Study the drawing (mm; zero at the part's minimum x, y, z) and answer. A direction names the side the tool comes from. Coordinates: 2 decimals unless noted, no trailing zeros. Write each loop counter-clockwise with the first axis right and the second up, starting at its lowest first coordinate (ties: lowest second). Pieces come first, ordered by that corner, then holes. Notation, with made-up numbers: (8.5, -19) -> (26.5, -19) arc R14 ccw to (26.5, -8) -> close; hole circle Ø7 at (-9.75, 20). An arc over 180 degrees is marked (long way). Write each question's results on one line, items separated by ' | '. Start each with the question number.
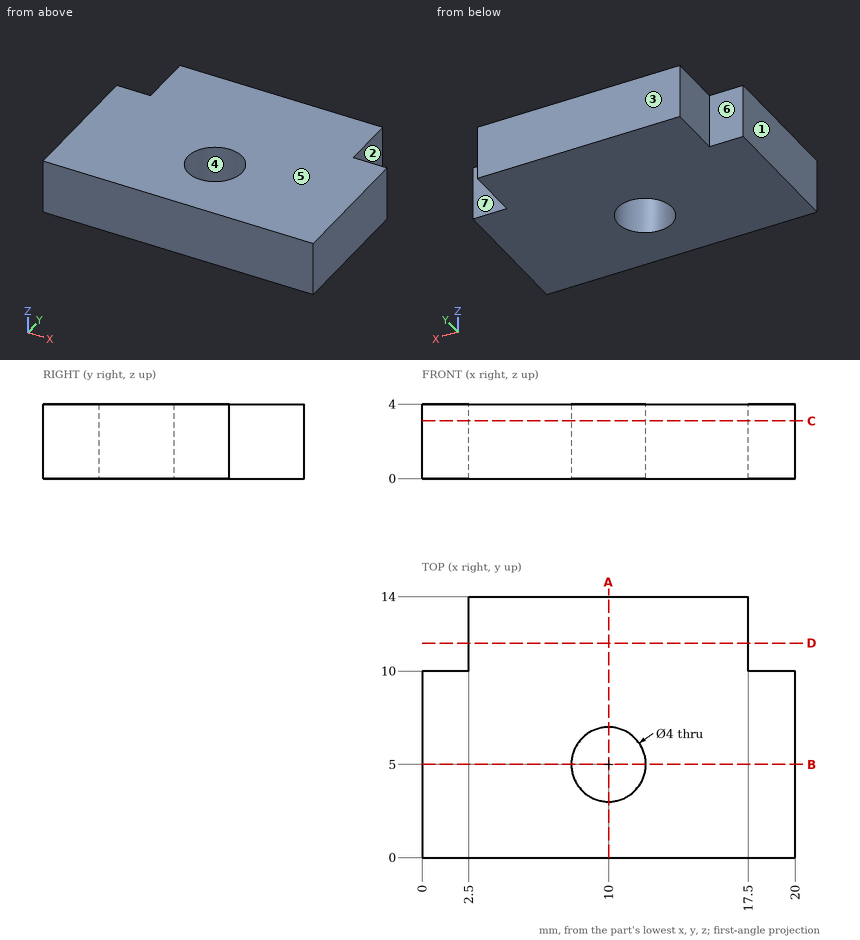
1. Given pin 1 Ø2 at (y, z) = (12.5, 2) entering from +X; pin 2 Ø1 at (x, z) = (13, 2.5) entering from -Y, each flat-ended and moving along its own axis, determine where each tip first touches the part or whether it passes through.
2. Find the intervals of material crossed by L1, parallel to Y at x = 10, z = 1.5; L2, parallel to X at y = 11.5, z = 1.95; L3, parallel to Y at x = 8.5, z = 3.35, in increasing order.
3. Find section A-A on x = 10. Give the vertices of the cut face in (y, z).
4. Find section C-C on z = 3.1. Give the vertices of the cut face in (x, y), and give its area (3 significant figures).
5. Find section D-D on y = 11.5. Give the vertices of the cut face in (x, z), and give its area (3 significant figures).
6. For the marked faces 5, 6 and 7, determine the directions among +Z, -Z, +X, -X, +Y, -Y from which every point of the face is accessible in a straight line to the end or side of a thin tool.
7. Find section B-B on y = 5. Give the vertices of the cut face in (x, z).
8. Determine the mould class of the marked faces 1, 2, 3 and 4 for opening direction X: pulls with the +X half, pulls with the -X half, needs draft (parallel to the pull), parting line crosses it, or undercut.
Ans:
1) pin 1: stops at x = 17.5 | pin 2: stops at y = 0
2) L1: y = 0 to 3, 7 to 14 | L2: x = 2.5 to 17.5 | L3: y = 0 to 3.68, 6.32 to 14
3) outline: (0, 0) -> (3, 0) -> (3, 4) -> (0, 4) -> close; (7, 0) -> (14, 0) -> (14, 4) -> (7, 4) -> close
4) outline: (0, 0) -> (20, 0) -> (20, 10) -> (17.5, 10) -> (17.5, 14) -> (2.5, 14) -> (2.5, 10) -> (0, 10) -> close; hole circle Ø4 at (10, 5) | area: 247 mm²
5) outline: (2.5, 0) -> (17.5, 0) -> (17.5, 4) -> (2.5, 4) -> close | area: 60.0 mm²
6) face 5: +Z, +X, -X, +Y, -Y | face 6: +Z, -Z, -X, +Y | face 7: +Z, -Z, +X, +Y
7) outline: (0, 0) -> (8, 0) -> (8, 4) -> (0, 4) -> close; (12, 0) -> (20, 0) -> (20, 4) -> (12, 4) -> close
8) face 1: pulls with the -X half | face 2: pulls with the +X half | face 3: needs draft | face 4: undercut
